The model under review builds one solid part; all positions refer to its coordinate system, in mm. A direction names the side the tool comes from. Give positions to 0.01 mm unless a question says otherwise; leave off trailing zeros. Loops run counter-clockwise (first coordinate to the right, second up) from the corner with the lowest first, then second, coordinate; pieces in that order, holes last. Notation, with made-up numbers: (43, 80.25) - (49, 80.25) arc R23 cw to (49, 119.25) - close; hole circle Ø9 at (13, 2.25). An arc over 180 degrees is marked (long way). Return JSON: item names as keys, results as strings. Group by question number.
from build123d import *

# Parameters (mm, degrees)
BOSS_EXTRUDE1_DEPTH     = 54
FILLET1_R               = 15
SKETCH2_W               = 32
SKETCH2_H               = 28
CUT_EXTRUDE1_DEPTH      = 445
SKETCH3_W               = 13.8
SKETCH3_H               = 16.5
BOSS_EXTRUDE2_DEPTH     = 5.5
SKETCH4_W               = 13.8
SKETCH4_H               = 3.5
BOSS_EXTRUDE3_DEPTH     = 4
SKETCH5_R               = 1
CUT_EXTRUDE2_DEPTH      = 1
SKETCH6_W               = 28
SKETCH6_H               = 14
CUT_EXTRUDE3_DEPTH      = 8
SKETCH7_W               = 14
SKETCH7_H               = 2
CUT_EXTRUDE4_DEPTH      = 30
CUT_EXTRUDE4_DEPTH_BACK = 3


with BuildPart() as part:
    # Sketch1 → Boss-Extrude1 (new body)
    with BuildSketch(Plane(origin=(0, 0, 0), x_dir=(1, 0, 0), z_dir=(0, 1, 0))):
        with BuildLine():
            Line((-97.5, -18.771444772), (97.5, -18.771444772))
            Line((97.5, -18.771444772), (97.5, -158.031444772))
            ThreePointArc((97.5, -158.031444772), (0, -185.688415193), (-97.5, -158.031444772))
            Line((-97.5, -158.031444772), (-97.5, -18.771444772))
        make_face()
    extrude(amount=BOSS_EXTRUDE1_DEPTH)

    # Fillet1
    fillet1_edges = [part.edges().sort_by_distance(p)[0] for p in [
        (0, 54, 185.688415193),
    ]]
    fillet(fillet1_edges, radius=FILLET1_R)

    # Sketch2 → Cut-Extrude1 (cut)
    with BuildSketch(Plane.ZY.offset(97.5)):
        with Locations((34.771444772, 14)):
            Rectangle(SKETCH2_W, SKETCH2_H)
    extrude(amount=-CUT_EXTRUDE1_DEPTH, mode=Mode.SUBTRACT)

    # Sketch3 → Boss-Extrude2 (add)
    with BuildSketch(Plane.XZ):
        with Locations((0, 151.498415193)):
            Rectangle(SKETCH3_W, SKETCH3_H)
    extrude(amount=BOSS_EXTRUDE2_DEPTH)

    # Sketch4 → Boss-Extrude3 (add)
    with BuildSketch(Plane(origin=(0, 0, 143.248415193), x_dir=(-1, 0, 0), z_dir=(0, 0, -1))):
        with Locations((0, -3.75)):
            Rectangle(SKETCH4_W, SKETCH4_H)
    extrude(amount=BOSS_EXTRUDE3_DEPTH)

    # Sketch5 → Cut-Extrude2 (cut)
    with BuildSketch(Plane(origin=(0, 54, 0), x_dir=(1, 0, 0), z_dir=(0, 1, 0))):
        with Locations((0, -43.438827689)):
            Circle(SKETCH5_R)
        with Locations((3, -43.438827689)):
            Circle(SKETCH5_R)
        with Locations((-3, -43.438827689)):
            Circle(SKETCH5_R)
    extrude(amount=-CUT_EXTRUDE2_DEPTH, mode=Mode.SUBTRACT)

    # Sketch6 → Cut-Extrude3 (cut)
    with BuildSketch(Plane(origin=(0, 54, 0), x_dir=(1, 0, 0), z_dir=(0, 1, 0))):
        with Locations((0, -59.925549651)):
            Rectangle(SKETCH6_W, SKETCH6_H)
    extrude(amount=-CUT_EXTRUDE3_DEPTH, mode=Mode.SUBTRACT)

    # Sketch7 → Cut-Extrude4 (cut, two sides)
    with BuildSketch(Plane(origin=(-14, 0, 0), x_dir=(0, 0, -1), z_dir=(1, 0, 0))) as cut_extrude4_sk:
        with Locations((-59.925549651, 47)):
            Rectangle(SKETCH7_W, SKETCH7_H)
    extrude(amount=CUT_EXTRUDE4_DEPTH, mode=Mode.SUBTRACT)
    extrude(cut_extrude4_sk.sketch, amount=-CUT_EXTRUDE4_DEPTH_BACK, mode=Mode.SUBTRACT)


solid = part.part
Item 1: Take a section at B-B (y = 15). State the section outline as (x, z) points, then the cut area to 3 significant figures.
Item 2: Take a section at A-A (z = 60.5). State the section outline as (x, y) points, then the cut area to 3 significant figures.
Item 3: Take a section at C-C (z = 120). State the section outline as (x, y) points.
Item 4: Mouldability with a two-part tool opening along X and no side actions: class faces 1 (the face through (-1, 50, 52.926)), 2 (the face through (-97.5, 27, 89)), 3 (the face through (-14, 51, 60)), 4 (the face through (6.9, -3, 150)) as +X half, -X half, draft (parallel to the pull), parting line (faces both ways), or undercut.
Item 5: For L1, parallel to Y at x = 58, z = 29.5; L2, parallel to Y at x = 37, z = 112; L3, parallel to Z at x = -35.5, y = 3.5, list the stretches that pass through material, from the lowest coordinate up. Write a range as from..to.
Item 6: Tool access review of faces 5 (the face through (14, 51, 60)), 6 (the face through (-1, 14, 50.771)), 7 (the face through (0, -3, 159.748)): name each direction out of +Z, -Z, +X, -X, +Y, -Y from which nothing blocks a thin tool from reaching the whole face with its end or side.
Item 7: For P1, Ø2.5, axis at x = -15.5, z = 61, coming from the -Y side; P2, Ø1.8, axis at x = -3, z = 43.44, coming from the -Y side; P3, Ø0.6, axis at x = 0, z = 43.5, coming from the +Y side, all flat-tipped, find the tip position at first contact; note any pin that passes through.
Check sheet entries:
{
 "1": {"outline": "(-97.5, 50.77) - (97.5, 50.77) - (97.5, 158.03) arc R185.69 ccw to (-97.5, 158.03) - close", "area": "24,600 mm^2"},
 "2": {"outline": "(-97.5, 0) - (97.5, 0) - (97.5, 54) - (14, 54) - (14, 48) - (16, 48) - (16, 46) - (-17, 46) - (-17, 48) - (-14, 48) - (-14, 54) - (-97.5, 54) - close", "area": "10,300 mm^2"},
 "3": {"outline": "(-97.5, 0) - (97.5, 0) - (97.5, 54) - (-97.5, 54) - close"},
 "4": {"face 1": "undercut", "face 2": "-X half", "face 3": "undercut", "face 4": "+X half"},
 "5": {"L1": "y = 28..54", "L2": "y = 0..54", "L3": "z = 50.77..182.26"},
 "6": {"face 5": "+Y", "face 6": "-Z, +X, -X, -Y", "face 7": "+Z, +X, -X, -Y"},
 "7": {"P1": "stops at y = 0", "P2": "stops at y = 28", "P3": "stops at y = 53"}
}
